Check sheet for the modelled part. Datum: model origin and axes. Units: mm. Round coordinates to 2 decimals unless told otherwise and drop trailing zeros. Loops run counter-clockwise (first coordinate to the right, second up) from the corner with the lowest first, then second, coordinate; pieces in that order, holes last. Notation, with made-up numbers: (87, 41.25) - (144, 41.25) arc R35 ccw to (144, 79.25) - close; hole circle Ø8 at (-18, -16). An arc over 180 degrees is marked (long way). Put each result on its own line as item: value.
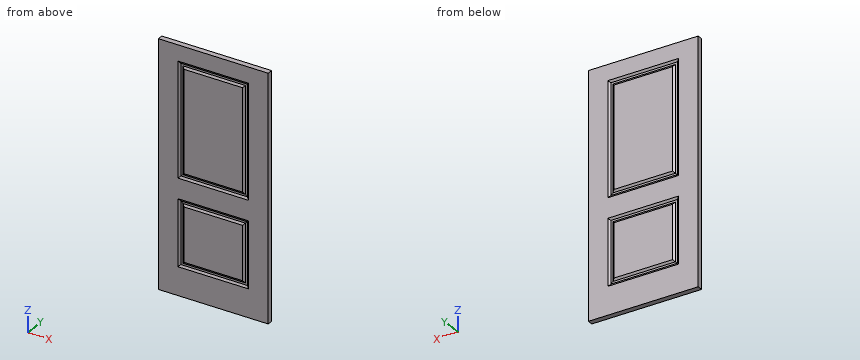
```python
from build123d import *

# Parameters (mm, degrees)
F0_W      = 907.25625
F0_H      = 44.45
F1_DEPTH  = 2012.95
F2_W      = 584.2
F2_H      = 546.1
F3_DEPTH  = 44.451
F8_DEPTH  = 939.8
F9_DEPTH  = 546.1
F11_DEPTH = 44.451
F13_DEPTH = 907.25625
F15_DEPTH = 44.4510000001
F17_W     = 482.6000000008
F17_H     = 44.4500000001
F18_DEPTH = 838.2
F19_W     = 482.6000000007
F19_H     = 44.45
F20_DEPTH = 444.5


with BuildPart() as f1:
    # F0 (on Top) → F1 (new body)
    with BuildSketch(Plane.XY):
        with Locations((-453.628125, 22.225)):
            Rectangle(F0_W, F0_H)
    extrude(amount=F1_DEPTH)

    # F2 (on Front) → F3 (cut, through all)
    with BuildSketch(Plane.XZ):
        Polygon((-745.728125, 1882.775), (-745.728125, 942.975), (-161.528125, 942.975), (-161.528125, 1882.775), (-453.628125, 1882.775), align=None)
        with Locations((-453.628125, 504.825)):
            Rectangle(F2_W, F2_H)
    extrude(amount=-F3_DEPTH, mode=Mode.SUBTRACT)

    # F6 (on face) → F8 (join, through all)
    with BuildSketch(Plane(origin=(0, 0, 1882.775), x_dir=(1, 0, 0), z_dir=(0, 0, -1))):
        Polygon((-694.928125, -22.225), (-694.928125, 0), (-712.3942085743, -10.8310357451), (-720.328125, -10.8310357451), (-728.2620414257, -10.8310357451), (-745.728125, 0), (-745.728125, -22.225), (-745.728125, -44.45), (-728.2620414257, -33.6189642549), (-720.328125, -33.6189642549), (-712.3942085743, -33.6189642549), (-694.928125, -44.45), align=None)
        Polygon((-212.328125, -22.225), (-212.328125, -44.45), (-194.8620414257, -33.6189642549), (-186.928125, -33.6189642549), (-178.9942085743, -33.6189642549), (-161.528125, -44.45), (-161.528125, -22.225), (-161.528125, 0), (-178.9942085743, -10.8310357451), (-186.928125, -10.8310357451), (-194.8620414257, -10.8310357451), (-212.328125, 0), align=None)
    extrude(amount=F8_DEPTH)

    # F7 (on face) → F9 (join, through all)
    with BuildSketch(Plane.XY.offset(231.775)):
        Polygon((-745.728125, 22.225), (-745.728125, 0), (-728.2620414257, 10.8310357451), (-720.328125, 10.8310357451), (-712.3942085743, 10.8310357451), (-694.928125, 0), (-694.928125, 22.225), (-694.928125, 44.45), (-712.3942085743, 33.6189642549), (-720.328125, 33.6189642549), (-728.2620414257, 33.6189642549), (-745.728125, 44.45), align=None)
        Polygon((-212.328125, 44.45), (-212.328125, 22.225), (-212.328125, 0), (-194.8620414257, 10.8310357451), (-186.928125, 10.8310357451), (-178.9942085743, 10.8310357451), (-161.528125, 0), (-161.528125, 22.225), (-161.528125, 44.45), (-178.9942085743, 33.6189642549), (-186.928125, 33.6189642549), (-194.8620414257, 33.6189642549), align=None)
    extrude(amount=F9_DEPTH)

    # F10 (on Front) → F11 (cut, through all)
    with BuildSketch(Plane.XZ):
        Polygon((-745.728125, 1882.775), (-453.628125, 1590.675), (-161.528125, 1882.775), (-212.328125, 1882.775), (-694.928125, 1882.775), align=None)
        Polygon((-161.528125, 942.975), (-453.628125, 1235.075), (-745.728125, 942.975), (-694.928125, 942.975), (-212.328125, 942.975), align=None)
        Polygon((-161.528125, 777.875), (-212.328125, 777.875), (-694.928125, 777.875), (-745.728125, 777.875), (-472.678125, 504.825), (-453.628125, 523.875), (-434.578125, 504.825), align=None)
        Polygon((-161.528125, 231.775), (-434.578125, 504.825), (-453.628125, 485.775), (-472.678125, 504.825), (-745.728125, 231.775), (-694.928125, 231.775), (-212.328125, 231.775), align=None)
        Polygon((-453.628125, 485.775), (-434.578125, 504.825), (-453.628125, 523.875), (-472.678125, 504.825), align=None)
    extrude(amount=-F11_DEPTH, mode=Mode.SUBTRACT)


with BuildPart() as f13:
    # F12 (on Right) → F13 (new body, through all)
    with BuildSketch(Plane.YZ):
        Polygon((44.45, 1882.775), (0, 1882.775), (10.8310357451, 1865.3089164258), (10.8310357451, 1849.4410835743), (0, 1831.975), (44.45, 1831.975), (33.6189642549, 1849.4410835743), (33.6189642549, 1865.3089164256), align=None)
    extrude(amount=-F13_DEPTH)


with BuildPart() as f13b:
    # F12 (on Right) → F13, piece 2 (new body, through all)
    with BuildSketch(Plane.YZ):
        Polygon((10.8310357452, 960.4410835743), (1e-10, 942.9750000002), (44.45, 942.975), (33.6189642548, 960.4410835744), (33.6189642549, 976.3089164258), (44.45, 993.775), (0, 993.775), (10.831035745, 976.308916426), align=None)
    extrude(amount=-F13_DEPTH)


with BuildPart() as f13c:
    # F12 (on Right) → F13, piece 3 (new body, through all)
    with BuildSketch(Plane.YZ):
        Polygon((33.6189642549, 744.5410835742), (33.6189642549, 760.4089164257), (44.4499999998, 777.8749999997), (0, 777.875), (10.831035745, 760.4089164259), (10.8310357451, 744.5410835743), (1e-10, 727.0750000001), (44.45, 727.075), align=None)
    extrude(amount=-F13_DEPTH)


with BuildPart() as f13d:
    # F12 (on Right) → F13, piece 4 (new body, through all)
    with BuildSketch(Plane.YZ):
        Polygon((44.45, 231.7749999998), (33.618964255, 249.241083574), (33.6189642549, 265.1089164257), (44.4499999999, 282.5749999998), (0, 282.575), (10.8310357451, 265.1089164258), (10.8310357451, 249.2410835743), (0, 231.7750000002), align=None)
    extrude(amount=-F13_DEPTH)


with BuildPart() as f15_tool:
    # F14 (on Front) → F15 (new body, through all)
    with BuildSketch(Plane.XZ):
        Polygon((-745.728125, 777.875), (-745.728125, 231.775), (-472.678125, 504.825), align=None)
        Polygon((-161.528125, 777.875), (-434.578125, 504.825), (-161.528125, 231.775), align=None)
        Polygon((-453.628125, 523.875), (-472.678125, 504.825), (-453.628125, 485.775), (-434.578125, 504.825), align=None)
        Polygon((-161.528125, 1882.775), (-453.628125, 1590.675), (-745.728125, 1882.775), (-745.728125, 942.975), (-453.628125, 1235.075), (-161.528125, 942.975), align=None)
    extrude(amount=-F15_DEPTH)


with BuildPart() as f13_1:
    add(f13.part)

    # F15: cut by f15_tool
    add(f15_tool.part, mode=Mode.SUBTRACT)


with BuildPart() as f13b_1:
    add(f13b.part)

    # F15: cut by f15_tool
    add(f15_tool.part, mode=Mode.SUBTRACT)


with BuildPart() as f13c_1:
    add(f13c.part)

    # F15: cut by f15_tool
    add(f15_tool.part, mode=Mode.SUBTRACT)


with BuildPart() as f13d_1:
    add(f13d.part)

    # F15: cut by f15_tool
    add(f15_tool.part, mode=Mode.SUBTRACT)


with BuildPart() as f1_1:
    add(f1.part)

    # F16: union F13, F13b, F13c, F13d
    add(f13_1.part)
    add(f13b_1.part)
    add(f13c_1.part)
    add(f13d_1.part)

    # F17 (on face) → F18 (join, through all)
    with BuildSketch(Plane.XY.offset(993.775)):
        with Locations((-453.6281250004, 22.2249999999)):
            Rectangle(F17_W, F17_H)
    extrude(amount=F18_DEPTH)

    # F19 (on face) → F20 (join, through all)
    with BuildSketch(Plane.XY.offset(282.575)):
        with Locations((-453.6281250003, 22.225)):
            Rectangle(F19_W, F19_H)
    extrude(amount=F20_DEPTH)


solid = f1_1.part
```
Item 1: Go/stop test with flat-tipped pins: pin 1 (5 mm diameter, centred on x = -479, z = 968, fed in from +Y); pin 2 (12.5 mm diameter, centred on x = -503.5, z = 753, fed in from -Y); pin 3 (17.5 mm diameter, centred on x = -435.5, z = 260, fed in from +Y). Record where each tip stops, or that it passes through.
Filled sheet:
pin 1: y = 33.62
pin 2: y = 10.83
pin 3: y = 35.88
Item 2: Section check A-A on z = 672. Enter the section's corners in (x, y).
Filled sheet:
outline: (-907.26, 0) - (-745.73, 0) - (-728.26, 10.83) - (-712.39, 10.83) - (-694.93, 0) - (-212.33, 0) - (-194.86, 10.83) - (-178.99, 10.83) - (-161.53, 0) - (0, 0) - (0, 44.45) - (-161.53, 44.45) - (-178.99, 33.62) - (-194.86, 33.62) - (-212.33, 44.45) - (-694.93, 44.45) - (-712.39, 33.62) - (-728.26, 33.62) - (-745.73, 44.45) - (-907.26, 44.45) - close
Item 3: Thickness scan on line 1 (Z direction, x = -371, y = 37.5); line 2 (X direction, y = 4, z = 513); line 3 (Z direction, x = -234.5, y = 4.5). Record the ranges inside material, lowest first. Write a range as from..to.
Filled sheet:
line 1: 0..242.98, 271.37..738.28, 766.67..954.18, 982.57..1843.18, 1871.57..2012.95
line 2: -907.26..-739.28, -701.38..-205.88, -167.98..0
line 3: 0..239.03, 275.32..734.33, 770.62..950.23, 986.52..1839.23, 1875.52..2012.95
